Part print with two shaded views. Sizes in mm from the minimum x, y, z corner. A direction names the side the tool comes from. Give positions to 0.01 mm unless a question says otherwise; leave off trailing zeros. Order: outer loops, then holes, each group sorted by start corner. A loop starts at its lowest first (then second) coordinate and runs counter-clockwise, first axis right, second up. Notation, with made-up numbers: (-4, 64.25) -> (33, 64.25) arc R13 cw to (33, 77.25) -> close; hole circle Ø10 at (20, -8). An arc over 180 degrees is marked (long way). Write item = value, one per line. Start each with the question number.
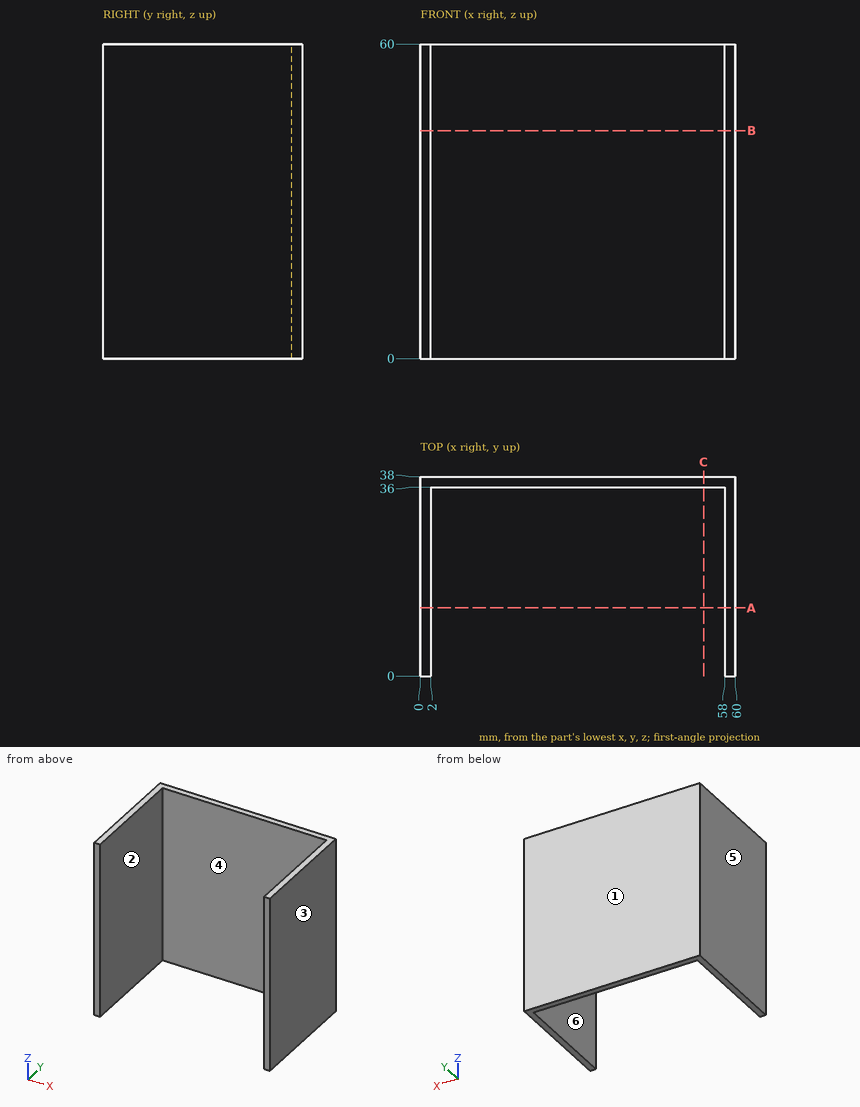
(1) Mould opens along X. For the marked faces 1, 2, 3 and 4 say: released by +X, released by -X, zero draft, split by the parting line, or undercut.
(2) Cut at B-B, the plane z = 43.5. Give the cut face in (x, y), plus the area to 3 significant figures.
(3) Flat gauge pin, fed straight in: P1, Ø2, axis at x = 49, z = 46, coming from the -Y side. Where does the tip first touch, or does it go through?
(4) Cut at C-C, the plane x = 54. Give the cut face in (y, z).
(5) Cut at A-A, the plane y = 13. Give the cut face in (x, z), plus the area to 3 significant figures.
(6) Wall check: line 1 (X direction, y = 21, z = 12); line 2 (Y direction, x = 23, z = 52). Give the ranges that are in metal, low to high. Write a range as [from, to].
(7) 3-axis set-ups, long thin cutter, end or side, ignore diameter. For the marked faces 5 and 6: which of +Z, -Z, +X, -X, +Y, -Y reach the whole face in a straight line?
Results:
q1.face_1 = zero draft
q1.face_2 = undercut
q1.face_3 = released by +X
q1.face_4 = undercut
q2.outline = (0, 0) -> (2, 0) -> (2, 36) -> (58, 36) -> (58, 0) -> (60, 0) -> (60, 38) -> (0, 38) -> close
q2.area = 264 mm2
q3.P1 = 36
q4.outline = (36, 0) -> (38, 0) -> (38, 60) -> (36, 60) -> close
q5.outline = (0, 0) -> (2, 0) -> (2, 60) -> (0, 60) -> close; (58, 0) -> (60, 0) -> (60, 60) -> (58, 60) -> close
q5.area = 240 mm2
q6.line_1 = [0, 2], [58, 60]
q6.line_2 = [36, 38]
q7.face_5 = +Z, -Z, -X, +Y, -Y
q7.face_6 = +Z, -Z, -Y
